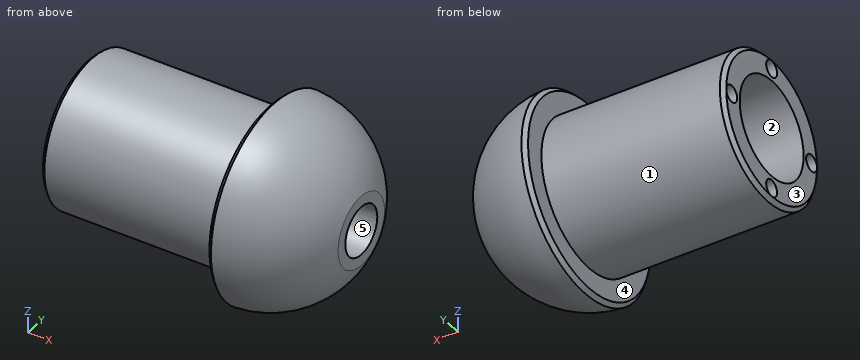
from build123d import *

# Parameters (mm, degrees)
F2_R      = 3.175
F3_DEPTH  = 15.24
F5_R      = 4.7625
F6_DEPTH  = 0.635
F7_R      = 6.35
F8_DEPTH  = 19.05
F10_R     = 1.0795
F11_DEPTH = 9.525


# Not quite as in the source:
# - a fillet or chamfer that OpenCascade refuses, or shapes differently, is made with other operations: its cross-section is extruded or revolved along the edge and cut away or added


with BuildPart() as f1:
    # F0 (on Front) → F1 (revolve)
    with BuildSketch(Plane.XZ):
        with BuildLine():
            Line((0, 9.525), (0, 0))
            Line((0, 0), (36.2827088845, 0))
            Line((36.2827088845, 0), (36.2827088845, 2.4049720118))
            ThreePointArc((36.2827088845, 2.4049720118), (31.8978835855, 9.7937006425), (23.8125, 12.7))
            Line((23.8125, 12.7), (23.8125, 9.525))
            Line((23.8125, 9.525), (0, 9.525))
        make_face()
    revolve(axis=Axis((18.1413544422, 0, 0), (-1, 0, 0)))

    # F2 (on face) → F3 (cut)
    with BuildSketch(Plane.YZ.offset(36.2827088845)):
        Circle(F2_R)
    extrude(amount=-F3_DEPTH, mode=Mode.SUBTRACT)

    # F5 (on offset) → F6 (cut)
    with BuildSketch(Plane.YZ.offset(36.2827088845)):
        Circle(F5_R)
    extrude(amount=-F6_DEPTH, mode=Mode.SUBTRACT)

    # F7 (on face) → F8 (cut)
    with BuildSketch(Plane(origin=(0, 0, 0), x_dir=(0, -1, 0), z_dir=(-1, 0, 0))):
        Circle(F7_R)
    extrude(amount=-F8_DEPTH, mode=Mode.SUBTRACT)

    # F9: chamfer of 0.508 on 2 edges, made by hand

    # F9_s1 → F9_t2 (revolve, cut)
    with BuildSketch(Plane.XZ):
        with BuildLine():
            Line((23.8125, 12.1814120692), (24.3416666667, 12.6889709054))
            ThreePointArc((24.3416666667, 12.6889709054), (24.0843208941, 12.6970907456), (23.8125, 12.7))
            Line((23.8125, 12.7), (23.8125, 12.1814120692))
        make_face()
    revolve(axis=Axis((23.8125, 0, 0), (-1, 0, 0)), mode=Mode.SUBTRACT)

    # F9_s3 → F9_t4 (revolve, cut)
    with BuildSketch(Plane.XZ):
        Polygon((0, 9.017), (0.508, 9.525), (0, 9.525), align=None)
    revolve(axis=Axis((0, 0, 0), (-1, 0, 0)), mode=Mode.SUBTRACT)

    # F10 (on face) → F11 (cut)
    with BuildSketch(Plane(origin=(0, 0, 0), x_dir=(0, -1, 0), z_dir=(-1, 0, 0))):
        with Locations((0, 7.9375)):
            Circle(F10_R)
        with Locations((0, -7.9375)):
            Circle(F10_R)
        with Locations((7.9375, 0)):
            Circle(F10_R)
        with Locations((-7.9375, 0)):
            Circle(F10_R)
    extrude(amount=-F11_DEPTH, mode=Mode.SUBTRACT)


solid = f1.part
Geometry: final body of the model. Coordinates: model frame, mm. Face numbers are marked on the shaded views. A direction names the side the tool comes from. Give positions to 0.01 mm unless a question says otherwise; leave off trailing zeros. Write each loop counter-clockwise with the first axis right and the second up, starting at its lowest first coordinate (ties: lowest second). Pieces come first, ordered by that corner, then holes. Notation, with made-up numbers: M 62,30.5 L 92,30.5 A33 cw 92,67.5 Z; hole C 73,64 d8. An arc over 180 degrees is marked long. Answer in a Markdown table with one row per item. Add a question column.
(1) Section A-A on x = 10. Return loops of the section in (y, z) (3 decimals), and give its area (3 significant figures).
(2) Mould query, pull axis Z, two halves, no side actions, for the marked faces 1, 2 and 3. Classes: +Z half, -Z half, draft (parallel to the pull), parting line (faces both ways), or undercut.
(3) Ray query, line 1 (Y direction, x = 16.5, z = -0.25); line 2 (X direction, y = -2, z = 2.5); line 3 (Z direction, x = 28.5, y = 1.75). Return the intervals inside material, ascending.
(4) Reachability of the marked faces 4 and 5 from +Z, -Z, +X, -X, +Y, -Y: full face, straight path, thin tool, end or side. Return the list, or none.
(5) Section B-B on x = 22. Return loops of the section in (y, z) (3 decimals).
(6) First-contact query: pin 1 (4 mm diameter, centred on y = 7, z = 7, fed in from +X); pin 2 (3.5 mm diameter, centred on y = -7.94, z = 0, fed in from +X); pin 3 (2 mm diameter, centred on x = 26, y = 5, fed in from +Z); pin 4 (10 mm diameter, centred on y = 3.5, z = -4, fed in from +X). Flat tips, straight axial feed; report the tip coordinate or a pass-through.
Result set:
| question | item | result |
|---|---|---|
| 1 | outline | C 0,0 d19.05; hole C 0,0 d12.7 |
| 1 | area | 158 mm^2 |
| 2 | face 1 | parting line |
| 2 | face 2 | undercut |
| 2 | face 3 | draft |
| 3 | line 1 | y = -9.52 to -6.35, 6.35 to 9.52 |
| 3 | line 2 | x = 19.05 to 35.65 |
| 3 | line 3 | z = -11.67 to -2.65, 2.65 to 11.67 |
| 4 | face 4 | -X |
| 4 | face 5 | +X |
| 5 | outline | C 0,0 d19.05; hole C 0,0 d6.35 |
| 6 | pin 1 | stops at x = 33.76 |
| 6 | pin 2 | stops at x = 34.9 |
| 6 | pin 3 | stops at z = 11.89 |
| 6 | pin 4 | stops at x = 35.65 |
